Model file for the job. Use its own axes, mm. A direction names the side the tool comes from. Give positions to 0.01 mm unless a question says otherwise; leave off trailing zeros. Loops run counter-clockwise (first coordinate to the right, second up) from the corner with the lowest first, then second, coordinate; pieces in that order, holes last. Notation, with made-up numbers: M -32,26 L -8,26 A12 cw -8,37 Z; hole C 27,-20 d11. An arc over 180 degrees is marked long. Answer in a Markdown table with one row per item.
```python
from build123d import *

# Parameters (mm, degrees)
SKETCH1_W               = 40
SKETCH1_H               = 10
SKETCH1_R               = 1.5
SKETCH1_W_2             = 15
SKETCH1_H_2             = 6
BOSS_EXTRUDE1_DEPTH     = 6
SKETCH1_3_W             = 15
SKETCH1_3_H             = 6
BOSS_EXTRUDE2_DEPTH     = 4
BOSS_EXTRUDE3_START     = -2.5
SKETCH2_R               = 1.75
SKETCH2_R_2             = 11.5
BOSS_EXTRUDE3_DEPTH     = 5
SKETCH3_W               = 40
SKETCH3_H               = 6
CUT_EXTRUDE1_DEPTH      = 0.5
BOSS_EXTRUDE4_START     = -7.5
SKETCH2_3_R             = 1.75
SKETCH2_3_R_2           = 11.5
BOSS_EXTRUDE4_DEPTH     = 2
SKETCH4_R               = 1.25
BOSS_EXTRUDE5_DEPTH     = 7
BOSS_EXTRUDE6_START     = 2.4
SKETCH4_3_R             = 1.25
BOSS_EXTRUDE6_DEPTH     = 2.4
SKETCH5_R               = 2.902241855
SKETCH5_R_2             = 1.35
SKETCH5_R_3             = 2.755762568
BOSS_EXTRUDE7_DEPTH     = 6
CUT_EXTRUDE2_DEPTH      = 69.628757271
CUT_EXTRUDE2_DEPTH_BACK = 16
SKETCH5_2_R             = 1.35


with BuildPart() as part:
    # Sketch1 → Boss-Extrude1 (new body)
    with BuildSketch(Plane.XY):
        with Locations((20, 5)):
            Rectangle(SKETCH1_W, SKETCH1_H)
        with Locations((5, 5)):
            Circle(SKETCH1_R, mode=Mode.SUBTRACT)
        with Locations((35, 5)):
            Circle(SKETCH1_R, mode=Mode.SUBTRACT)
        with Locations((20, 5)):
            Rectangle(SKETCH1_W_2, SKETCH1_H_2, mode=Mode.SUBTRACT)
    extrude(amount=BOSS_EXTRUDE1_DEPTH)

    # Sketch1<3> → Boss-Extrude2 (add)
    with BuildSketch(Plane.XY):
        with Locations((20, 5)):
            Rectangle(SKETCH1_3_W, SKETCH1_3_H)
    extrude(amount=BOSS_EXTRUDE2_DEPTH)

    # Sketch2 → Boss-Extrude3 (add)
    # profile 1 of 2: a face of its own
    with BuildSketch(Plane(origin=(0, 10, 0), x_dir=(1, 0, 0), z_dir=(0, 1, 0)).offset(BOSS_EXTRUDE3_START)):
        with BuildLine():
            Line((0, 0), (8, 0))
            Line((8, 0), (8, 12.1))
            ThreePointArc((8, 12.1), (20, 24.1), (32, 12.1))
            Line((32, 12.1), (32, 0))
            Line((32, 0), (40, 0))
            Line((40, 0), (49.920310217, 12.1))
            Line((49.920310217, 12.1), (25.291502622, 40.020310217))
            Line((25.291502622, 40.020310217), (14.708497378, 40.020310217))
            Line((14.708497378, 40.020310217), (-9.920310217, 12.1))
            Line((-9.920310217, 12.1), (0, 0))
        make_face()
        with Locations(Location((-1.920310217, 12.1, 0), (0, 0, 270))):
            Circle(SKETCH2_R, mode=Mode.SUBTRACT)
        with Locations(Location((41.920310217, 12.1, 0), (0, 0, 270))):
            Circle(SKETCH2_R, mode=Mode.SUBTRACT)
        with Locations(Location((20, 34.020310217, 0), (0, 0, 270))):
            Circle(SKETCH2_R, mode=Mode.SUBTRACT)
    # profile 2 of 2: a face of its own
    with BuildSketch(Plane(origin=(0, 10, 0), x_dir=(1, 0, 0), z_dir=(0, 1, 0)).offset(BOSS_EXTRUDE3_START)):
        with BuildLine():
            Line((8, 12.1), (8, 0))
            Line((8, 0), (32, 0))
            Line((32, 0), (32, 12.1))
            ThreePointArc((32, 12.1), (20, 24.1), (8, 12.1))
        make_face()
        with Locations(Location((20, 12.1, 0), (0, 0, 270))):
            Circle(SKETCH2_R_2, mode=Mode.SUBTRACT)
    extrude(amount=-BOSS_EXTRUDE3_DEPTH)

    # Sketch3 → Cut-Extrude1 (cut)
    with BuildSketch(Plane(origin=(0, 0, 0), x_dir=(1, 0, 0), z_dir=(0, 1, 0))):
        with Locations((20, -3)):
            Rectangle(SKETCH3_W, SKETCH3_H)
    extrude(amount=CUT_EXTRUDE1_DEPTH, mode=Mode.SUBTRACT)

    # Sketch2<3> → Boss-Extrude4 (add)
    # profile 1 of 2: a face of its own
    with BuildSketch(Plane(origin=(0, 10, 0), x_dir=(1, 0, 0), z_dir=(0, 1, 0)).offset(BOSS_EXTRUDE4_START)):
        with BuildLine():
            Line((0, 0), (8, 0))
            Line((8, 0), (8, 12.1))
            ThreePointArc((8, 12.1), (20, 24.1), (32, 12.1))
            Line((32, 12.1), (32, 0))
            Line((32, 0), (40, 0))
            Line((40, 0), (49.920310217, 12.1))
            Line((49.920310217, 12.1), (25.291502622, 40.020310217))
            Line((25.291502622, 40.020310217), (14.708497378, 40.020310217))
            Line((14.708497378, 40.020310217), (-9.920310217, 12.1))
            Line((-9.920310217, 12.1), (0, 0))
        make_face()
        with Locations(Location((-1.920310217, 12.1, 0), (0, 0, 270))):
            Circle(SKETCH2_3_R, mode=Mode.SUBTRACT)
        with Locations(Location((41.920310217, 12.1, 0), (0, 0, 270))):
            Circle(SKETCH2_3_R, mode=Mode.SUBTRACT)
        with Locations(Location((20, 34.020310217, 0), (0, 0, 270))):
            Circle(SKETCH2_3_R, mode=Mode.SUBTRACT)
    # profile 2 of 2: a face of its own
    with BuildSketch(Plane(origin=(0, 10, 0), x_dir=(1, 0, 0), z_dir=(0, 1, 0)).offset(BOSS_EXTRUDE4_START)):
        with BuildLine():
            Line((8, 12.1), (8, 0))
            Line((8, 0), (32, 0))
            Line((32, 0), (32, 12.1))
            ThreePointArc((32, 12.1), (20, 24.1), (8, 12.1))
        make_face()
        with Locations(Location((20, 12.1, 0), (0, 0, 270))):
            Circle(SKETCH2_3_R_2, mode=Mode.SUBTRACT)
    extrude(amount=-BOSS_EXTRUDE4_DEPTH)

    # Sketch4 → Boss-Extrude5 (add)
    with BuildSketch(Plane(origin=(0, 7.5, 0), x_dir=(1, 0, 0), z_dir=(0, 1, 0))):
        Polygon((-25.886515965, -6), (-24.891502622, -6), (-24.891502622, 6), (-15.301186187, 6), (-4.919162091, 6), (4.919162091, -6), align=None)
        with Locations(Location((-21.891502622, -3.5, 0), (0, 0, 270))):
            Circle(SKETCH4_R, mode=Mode.SUBTRACT)
        with Locations(Location((-12.291502622, -3.5, 0), (0, 0, 270))):
            Circle(SKETCH4_R, mode=Mode.SUBTRACT)
    extrude(amount=-BOSS_EXTRUDE5_DEPTH)

    # Sketch4<3> → Boss-Extrude6 (add)
    with BuildSketch(Plane(origin=(0, 7.5, 0), x_dir=(1, 0, 0), z_dir=(0, 1, 0)).offset(BOSS_EXTRUDE6_START)):
        Polygon((-24.891502622, 6), (-24.891502622, -6), (4.919162091, -6), (0, 0), (-4.919162091, 6), (-15.301186187, 6), align=None)
        with Locations(Location((-21.891502622, -3.5, 0), (0, 0, 270))):
            Circle(SKETCH4_3_R, mode=Mode.SUBTRACT)
        with Locations(Location((-12.291502622, -3.5, 0), (0, 0, 270))):
            Circle(SKETCH4_3_R, mode=Mode.SUBTRACT)
    extrude(amount=-BOSS_EXTRUDE6_DEPTH)

    # Sketch5 → Boss-Extrude7 (add)
    # profile 1 of 2: a face of its own
    with BuildSketch(Plane.XY.offset(6)):
        with Locations((4.919162091, 5)):
            Circle(SKETCH5_R)
        with Locations(Location((4.919162091, 5, 0), (0, 0, 90))):
            Circle(SKETCH5_R_2, mode=Mode.SUBTRACT)
    # profile 2 of 2: a face of its own
    with BuildSketch(Plane.XY.offset(6)):
        with Locations((35, 5)):
            Circle(SKETCH5_R_3)
        with Locations((35, 5)):
            Circle(SKETCH5_R_2, mode=Mode.SUBTRACT)
    extrude(amount=-BOSS_EXTRUDE7_DEPTH)

    # Sketch5<2> → Cut-Extrude2 (cut, two sides: drawn at the far end of the back side and taken through both)
    with BuildSketch(Plane.XY.offset(6).offset(-CUT_EXTRUDE2_DEPTH_BACK)):
        with BuildLine():
            ThreePointArc((4.919162091, 3.65), (5.873756246, 4.045405845), (6.269162091, 5))
            ThreePointArc((6.269162091, 5), (5.873756246, 5.954594155), (4.919162091, 6.35))
            Line((4.919162091, 6.35), (4.919162091, 3.65))
        make_face()
        with BuildLine():
            Line((4.919162091, 3.65), (4.919162091, 6.35))
            ThreePointArc((4.919162091, 6.35), (3.569162091, 5), (4.919162091, 3.65))
        make_face()
        with Locations((35, 5)):
            Circle(SKETCH5_2_R)
    extrude(amount=CUT_EXTRUDE2_DEPTH + CUT_EXTRUDE2_DEPTH_BACK, mode=Mode.SUBTRACT)


solid = part.part
```
Q1. 3-axis set-ups, long thin cutter, end or side, ignore diameter. For faces 4 (the face through (-15, 5, -6)), 5 (the face through (35, 5, -10)), 6 (the face through (-13, 9.9, 0)), 7 (the face through (20, 9, 0)): which of +Z, -Z, +X, -X, +Y, -Y reach the whole face in a straight line?
Reported:
| item | result |
|---|---|
| face 4 | -X, +Y, -Y |
| face 5 | +Z |
| face 6 | +Z, -Z, -X, +Y |
| face 7 | -Z, +X, +Y |
Q2. Saw through at D-D (y = 8.75). Give the cut face in (x, z), and give its area (3 significant figures).
Reported:
| item | result |
|---|---|
| outline | M -24.89,-6 L -4.92,-6 L 0,0 L 40,0 L 40,6 L -24.89,6 Z; hole C -21.89,3.5 d2.5; hole C -12.29,3.5 d2.5 |
| area | 514 mm² |
Q3. Probe probe 1 along X at (y, z) = (4.25, -12.1); probe 2 along X at (y, z) = (3, 3.5); probe 3 along X at (y, z) = (7, -12.5). List the from-to ranges inside material, lowest first.
Reported:
| item | result |
|---|---|
| probe 1 | -9.92 to -3.67, -0.17 to 8.5, 31.5 to 40.17, 43.67 to 49.92 |
| probe 2 | -24.89 to -23.14, -20.64 to -13.54, -11.04 to 40 |
| probe 3 | -9.57 to -3.62, -0.22 to 8.51, 31.49 to 40.22, 43.62 to 49.57 |
Q4. Saw through at A-A (x = 20). Give the cut face in (y, z).
Reported:
| item | result |
|---|---|
| outline | M 0.5,-40.02 L 7.5,-40.02 L 7.5,-35.77 L 0.5,-35.77 Z; M 0.5,-32.27 L 7.5,-32.27 L 7.5,-23.6 L 0.5,-23.6 Z; M 0.5,-0.6 L 7.5,-0.6 L 7.5,0 L 10,0 L 10,6 L 8,6 L 8,4 L 2,4 L 2,6 L 0.5,6 Z |
Q5. Saw through at B-B (z = -17.5). Give the cut face in (x, y).
Reported:
| item | result |
|---|---|
| outline | M -5.16,0.5 L 9.85,0.5 L 9.85,7.5 L -5.16,7.5 Z; M 30.15,0.5 L 45.16,0.5 L 45.16,7.5 L 30.15,7.5 Z |
Q6. Drop flat-ended pins along their axis: pin 1 (5.5 mm diameter, centred on x = 20, z = -34.02, fed in from -Y); pin 2 (2 mm diameter, centred on y = 3.5, z = 5.5, fed in from +X); pin 3 (1 mm diameter, centred on x = 18.5, y = 3.5, fed in from +Z); pin 4 (3 mm diameter, centred on x = 41.92, z = -12.1, fed in from -Y). Give the stop position or say it passes through.
Reported:
| item | result |
|---|---|
| pin 1 | y = 0.5 |
| pin 2 | x = 40 |
| pin 3 | z = 4 |
| pin 4 | through |
Q7. Saw through at C-C (z = -2.5). Give the cut face in (x, y), and give its area (3 significant figures).
Reported:
| item | result |
|---|---|
| outline | M -24.89,0.5 L 13.67,0.5 L 13.67,7.5 L -2.05,7.5 L -2.05,9.9 L -24.89,9.9 Z; M 26.33,0.5 L 42.05,0.5 L 42.05,7.5 L 26.33,7.5 Z; hole C 4.92,5 d2.7; hole C 35,5 d2.7 |
| area | 423 mm² |
Q8. Mould opens along Y. For faces 1 (the face through (12.5, 5, 5)), 2 (the face through (13, 0.5, -22)), 3 (the face through (7, 5, 6)) say: released by +Y, released by -Y, zero draft, split by the parting line, or undercut.
Reported:
| item | result |
|---|---|
| face 1 | undercut |
| face 2 | released by -Y |
| face 3 | zero draft |
